The listing builds one solid part. Answer for the finished solid, in the listing's coordinates (mm). A direction names the side the tool comes from. Round coordinates to 2 decimals unless told otherwise and drop trailing zeros. Loops run counter-clockwise (first coordinate to the right, second up) from the corner with the lowest first, then second, coordinate; pieces in that order, holes last. Notation, with made-up numbers: (25, 14) - (72, 14) arc R9 ccw to (72, 27) - close; hole circle Ø2 at (77, 61). An arc over 180 degrees is marked (long way). One line per item, written item: value.
```python
from build123d import *

# Parameters (mm, degrees)
SKETCH1_R               = 0.508
SKETCH1_R_2             = 0.381
SKETCH1_R_3             = 1.016
BOSS_EXTRUDE1_DEPTH     = 1.905
BOSS_EXTRUDE2_START     = -1.524
SKETCH1_3_R             = 3.175
SKETCH1_3_R_2           = 1.016
BOSS_EXTRUDE2_DEPTH     = 1.524
CUT_EXTRUDE1_START      = -0.889
SKETCH2_R               = 2.158999876
SKETCH2_R_2             = 1.016
CUT_EXTRUDE1_DEPTH      = 0.889
SKETCH4_R               = 2.095500003
SKETCH4_R_2             = 1.016
CUT_EXTRUDE2_DEPTH      = 0.889
CUT_EXTRUDE3_DEPTH      = 19.858264168
CUT_EXTRUDE3_DEPTH_BACK = 19.858264168
SKETCH5_R               = 0.508


with BuildPart() as part:
    # Sketch1 → Boss-Extrude1 (new body)
    with BuildSketch(Plane.XY):
        with BuildLine():
            Line((17.659400579, 0.944821475), (0.402335264, 3.149404918))
            ThreePointArc((0.402335264, 3.149404918), (-3.175, 0), (0.402335264, -3.149404918))
            Line((0.402335264, -3.149404918), (17.659400579, -0.944821475))
            ThreePointArc((17.659400579, -0.944821475), (18.4912, 0), (17.659400579, 0.944821475))
        make_face()
        with Locations((16.891, 0)):
            Circle(SKETCH1_R, mode=Mode.SUBTRACT)
        with Locations((4.699, 0)):
            Circle(SKETCH1_R_2, mode=Mode.SUBTRACT)
        with Locations((6.985, 0)):
            Circle(SKETCH1_R, mode=Mode.SUBTRACT)
        with Locations((10.287, 0)):
            Circle(SKETCH1_R, mode=Mode.SUBTRACT)
        with Locations((13.589, 0)):
            Circle(SKETCH1_R, mode=Mode.SUBTRACT)
        Circle(SKETCH1_R_3, mode=Mode.SUBTRACT)
    extrude(amount=BOSS_EXTRUDE1_DEPTH)

    # Sketch1<3> → Boss-Extrude2 (add)
    with BuildSketch(Plane.XY.offset(BOSS_EXTRUDE2_START)):
        with Locations(Location((0, 0, 0), (0, 0, 82.719918909))):
            Circle(SKETCH1_3_R)
        Circle(SKETCH1_3_R_2, mode=Mode.SUBTRACT)
    extrude(amount=BOSS_EXTRUDE2_DEPTH)

    # Sketch2 → Cut-Extrude1 (cut)
    with BuildSketch(Plane.XY.offset(1.905).offset(CUT_EXTRUDE1_START)):
        Circle(SKETCH2_R)
        Circle(SKETCH2_R_2, mode=Mode.SUBTRACT)
    extrude(amount=CUT_EXTRUDE1_DEPTH, mode=Mode.SUBTRACT)

    # Sketch4 → Cut-Extrude2 (cut)
    with BuildSketch(Plane(origin=(0, 0, -1.524), x_dir=(-1, 0, 0), z_dir=(0, 0, -1))):
        Circle(SKETCH4_R)
        Circle(SKETCH4_R_2, mode=Mode.SUBTRACT)
    extrude(amount=-CUT_EXTRUDE2_DEPTH, mode=Mode.SUBTRACT)

    # Sketch5 → Cut-Extrude3 (cut, two sides: drawn at the far end of the back side and taken through both)
    # profile 1 of 2: a face of its own
    with BuildSketch(Plane(origin=(0, 0, 0), x_dir=(-1, 0, 0), z_dir=(0, 0, -1)).offset(-CUT_EXTRUDE3_DEPTH_BACK)):
        with BuildLine():
            Line((-17.659400579, -0.944821475), (-14, -1.412308489))
            Line((-14, -1.412308489), (-14, -0.29856825))
            ThreePointArc((-14, -0.29856825), (-14.097, 0), (-14, 0.29856825))
            Line((-14, 0.29856825), (-14, 1.412308489))
            Line((-14, 1.412308489), (-17.659400579, 0.944821475))
            ThreePointArc((-17.659400579, 0.944821475), (-18.4912, 0), (-17.659400579, -0.944821475))
        make_face()
        with Locations((-16.891, 0)):
            Circle(SKETCH5_R, mode=Mode.SUBTRACT)
    # profile 2 of 2: a face of its own
    with BuildSketch(Plane(origin=(0, 0, 0), x_dir=(-1, 0, 0), z_dir=(0, 0, -1)).offset(-CUT_EXTRUDE3_DEPTH_BACK)):
        with Locations((-16.891, 0)):
            Circle(SKETCH5_R)
    extrude(amount=CUT_EXTRUDE3_DEPTH + CUT_EXTRUDE3_DEPTH_BACK, mode=Mode.SUBTRACT)


solid = part.part
```
1) For a pull along Y with two mould halves and no side action, classify faces 1 (the flat face through (7.3, 2.27, 0.94)), 2 (the cylindrical face through (6.477, 0.022, 0.939)), 3 (the flat face through (14, -1, 1)) as released by +Y, released by -Y, zero draft, split by the parting line, or undercut.
Final values:
face 1: released by +Y
face 2: undercut
face 3: zero draft
2) A cutting plane is placed at B-B on z = 0.7. Give the vertices of the cut face in (x, y) (3 decimals).
Final values:
outline: (0.402, -3.149) - (14, -1.412) - (14, -0.299) arc R0.508 cw (long way) to (14, 0.299) - (14, 1.412) - (0.402, 3.149) arc R3.175 ccw (long way) to start; hole circle Ø2.032 at (0, 0); hole circle Ø0.762 at (4.699, 0); hole circle Ø1.016 at (6.985, 0); hole circle Ø1.016 at (10.287, 0)
3) Consider L1, parallel to Y at x = 0, z = 1.3 (3 decimals); L2, parallel to Z at x = 5.5, y = 0.5 (3 decimals); L3, parallel to Y at x = 0, z = 0.35 (3 decimals). Determine where each line is inside the solid, lowest interval first.
Final values:
L1: -3.175 to -2.159, 2.159 to 3.175
L2: 0 to 1.905
L3: -3.175 to -1.016, 1.016 to 3.175
4) Each of these flat-tipped pins is pushed along its axis until it touches: pin 1 Ø2 at (x, y) = (5, -2) entering from -Z; pin 2 Ø1.5 at (y, z) = (2.5, 1) entering from -X. Where does it stop, or does it pass through?
Final values:
pin 1: z = 0
pin 2: x = -2.65
5) A cutting plane is placed at A-A on x = 0. Give the vertices of the cut face in (y, z) (1 decimal).
Final values:
outline: (-3.2, -1.5) - (-2.1, -1.5) - (-2.1, -0.6) - (-1, -0.6) - (-1, 1) - (-2.2, 1) - (-2.2, 1.9) - (-3.2, 1.9) - close; (1, -0.6) - (2.1, -0.6) - (2.1, -1.5) - (3.2, -1.5) - (3.2, 1.9) - (2.2, 1.9) - (2.2, 1) - (1, 1) - close
6) A cutting plane is placed at C-C on y = 0. Give the number of separate pieces and of enclosed holes in the cut face, and give its area (3 significant figures).
Final values:
separate pieces: 5
enclosed holes: 0
area: 24.4 mm2
7) A cutting plane is placed at D-D on x = 7.25. Give the vertices of the cut face in (y, z) (3 decimals), and give its area (3 significant figures).
Final values:
outline: (-2.275, 0) - (-0.433, 0) - (-0.433, 1.905) - (-2.275, 1.905) - close; (0.433, 0) - (2.275, 0) - (2.275, 1.905) - (0.433, 1.905) - close
area: 7.02 mm2
8) For faces 4 (the cylindrical face through (1.16, 1.82, 1.45)), 5 (the flat face through (7.106, -2.293, 0.939)), 6 (the cylindrical face through (-1.127, 1.767, -1.086)), determine the directions among +Z, -Z, +X, -X, +Y, -Y from which every point of the face is accessible in a straight line to the end or side of a thin tool.
Final values:
face 4: +Z
face 5: +Z, -Z, +X, -Y
face 6: -Z
